```python
from build123d import *

# Parameters (mm, degrees)
SKETCH1_R           = 3.175
BOSS_EXTRUDE1_DEPTH = 15
SKETCH2_R           = 3.175
CUT_EXTRUDE1_DEPTH  = 15


with BuildPart() as part:
    # Sketch1 → Boss-Extrude1 (new body)
    with BuildSketch(Plane.XY):
        with BuildLine():
            Line((-10, 0), (-10, -25.4))
            Line((-10, -25.4), (10, -25.4))
            Line((10, -25.4), (10, 0))
            ThreePointArc((10, 0), (0, 10), (-10, 0))
        make_face()
        Circle(SKETCH1_R, mode=Mode.SUBTRACT)
    extrude(amount=BOSS_EXTRUDE1_DEPTH)

    # Sketch2 → Cut-Extrude1 (cut)
    with BuildSketch(Plane.XZ.offset(25.4)):
        with Locations(Location((0, 7.5, 0), (0, 0, 270))):
            Circle(SKETCH2_R)
    extrude(amount=-CUT_EXTRUDE1_DEPTH, mode=Mode.SUBTRACT)


solid = part.part
```
Geometry: final body of the model. Coordinates: model frame, mm. A direction names the side the tool comes from. Round coordinates to 2 decimals unless told otherwise and drop trailing zeros. Write each loop counter-clockwise with the first axis right and the second up, starting at its lowest first coordinate (ties: lowest second). Pieces come first, ordered by that corner, then holes.
Item 1: Section query D-D (z = 7.5). Return loops of the section in (x, y) (3 decimals).
Item 2: Material intervals for L1, parallel to Y at x = 0, z = 8.5 (3 decimals); L2, parallel to X at y = -17.25, z = 7.5 (3 decimals); L3, parallel to X at y = 0.5, z = 14, sorted ascending.
Item 3: Mould query, pull axis Z, two halves, no side actions, for faces 1 (the face through (-0.69, -3.1, 7.4)), 2 (the face through (0, -7, 0)), 3 (the face through (0, -10.4, 8)). Classes: +Z half, -Z half, draft (parallel to the pull), parting line (faces both ways), or undercut.
Item 4: Set-up query: faces 4 (the face through (0, 10, 7)), 5 (the face through (-1.93, -18, 10.02)). Return all of +Z, -Z, +X, -X, +Y, -Y with unobstructed straight access to the full face (end or side cutting, diameter ignored); none if empty.
Item 5: Section query A-A (x = 0). Return loops of the section in (y, z) (3 decimals), plus the area to 4 significant figures.
Item 6: Section query B-B (z = 3.5). Return loops of the section in (x, y) (3 decimals), plus the area to 3 significant figures.
Item 7: Pin query (flat end, axial travel): P1, Ø5, axis at x = 3, z = 7, coming from the +Y side; P2, Ø5, axis at x = 0, y = 0, coming from the +Z side. Return the tip coordinate at first contact, or that it passes through.
Item 8: Section query C-C (y = -16). Return loops of the section in (x, z) (3 decimals).
Completed:
1. outline: (-10, -25.4) - (-3.175, -25.4) - (-3.175, -10.4) - (3.175, -10.4) - (3.175, -25.4) - (10, -25.4) - (10, 0) arc R10 ccw to (-10, 0) - close; hole circle Ø6.35 at (0, 0)
2. L1: y = -10.4 to -3.175, 3.175 to 10
2. L2: x = -10 to -3.175, 3.175 to 10
2. L3: x = -9.99 to -3.14, 3.14 to 9.99
3. face 1: draft
3. face 2: -Z half
3. face 3: undercut
4. face 4: +Z, -Z, +Y
4. face 5: -Y
5. outline: (-25.4, 0) - (-3.175, 0) - (-3.175, 15) - (-25.4, 15) - (-25.4, 10.675) - (-10.4, 10.675) - (-10.4, 4.325) - (-25.4, 4.325) - close; (3.175, 0) - (10, 0) - (10, 15) - (3.175, 15) - close
5. area: 340.5 mm2
6. outline: (-10, -25.4) - (10, -25.4) - (10, 0) arc R10 ccw to (-10, 0) - close; hole circle Ø6.35 at (0, 0)
6. area: 633 mm2
7. P1: stops at y = 9.99
7. P2: passes through
8. outline: (-10, 0) - (10, 0) - (10, 15) - (-10, 15) - close; hole circle Ø6.35 at (0, 7.5)
